from build123d import *

# Parameters (mm, degrees)
SKETCH1_W          = 661.58618
SKETCH1_H          = 260.35
BASE_FLANGE1_DEPTH = 3.175
EDGE_FLANGE1_DEPTH = 306.87772


# Sheet-metal steps are written as plain solids
with BuildPart() as part:
    # Sketch1 → Base-Flange1 (new body)
    with BuildSketch(Plane(origin=(0, 0, 0), x_dir=(0, 0, -1), z_dir=(1, 0, 0))):
        Rectangle(SKETCH1_W, SKETCH1_H)
    extrude(amount=-BASE_FLANGE1_DEPTH)

    # Edge-Flange1 section (across the edge) → Edge-Flange1 (add)
    with BuildSketch(Plane(origin=(-3.175, -133.35, -153.43886), x_dir=(0, 1, 0), z_dir=(0, 0, 1))):
        with BuildLine():
            Line((-3.175, 3.175), (-3.175, 22.225))
            Line((-3.175, 22.225), (0, 22.225))
            Line((0, 22.225), (0, 3.175))
            ThreePointArc((0, 3.175), (0.92993597, 0.92993597), (3.175, 0))
            Line((3.175, 0), (3.175, -3.175))
            ThreePointArc((3.175, -3.175), (-1.315128061, -1.315128061), (-3.175, 3.175))
        make_face()
    extrude(amount=EDGE_FLANGE1_DEPTH)


solid = part.part
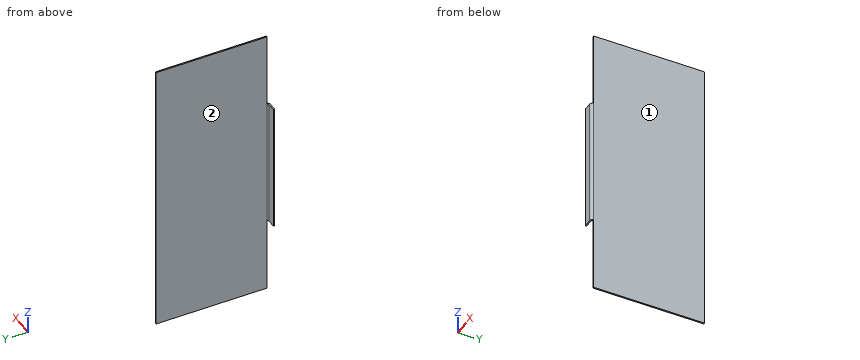
Verification items for the finished model (mm, model axes). Face numbers are marked on the shaded views. A direction names the side the tool comes from. Give positions to 0.01 mm unless a question says otherwise; leave off trailing zeros. Loops run counter-clockwise (first coordinate to the right, second up) from the corner with the lowest first, then second, coordinate; pieces in that order, holes last.
1. Go/stop test with flat-tipped pins: P1, Ø3.5, axis at x = -2, z = 272.5, coming from the -Y side (3 decimals); P2, Ø5.5, axis at x = -17.5, z = 11.5, coming from the +Y side; P3, Ø1.9, axis at x = -9, y = -132.5, coming from the +Z side. Record where each tip stops, or that it passes through.
Derived:
P1: stops at y = -130.175
P2: stops at y = -133.35
P3: stops at z = 153.44
2. Tool access check on the marked faces 1 and 2. Record the directions out of +Z, -Z, +X, -X, +Y, -Y that give a thin tool (end or side, any length) a straight path to the whole face; none if there is none.
Derived:
face 1: +Z, -Z, +X, +Y, -Y
face 2: +Z, -Z, -X, +Y
3. Cross-section at B-B on x = -12.5. Record the cut outline in (y, z) (3 decimals).
Derived:
outline: (-136.525, -153.439) - (-133.35, -153.439) - (-133.35, 153.439) - (-136.525, 153.439) - close
4. Cross-section at A-A on y = -95. Record the cut outline in (x, z) (3 decimals).
Derived:
outline: (-3.175, -330.793) - (0, -330.793) - (0, 330.793) - (-3.175, 330.793) - close
5. Material ranges on probe 1 along X at (y, z) = (86, -24.5) (3 decimals); probe 2 along Y at (x, z) = (-14.25, -76.5) (3 decimals); probe 3 along Y at (x, z) = (-0.75, -262) (3 decimals), recorded low to high.
Derived:
probe 1: x = -3.175 to 0
probe 2: y = -136.525 to -133.35
probe 3: y = -130.175 to 130.175
